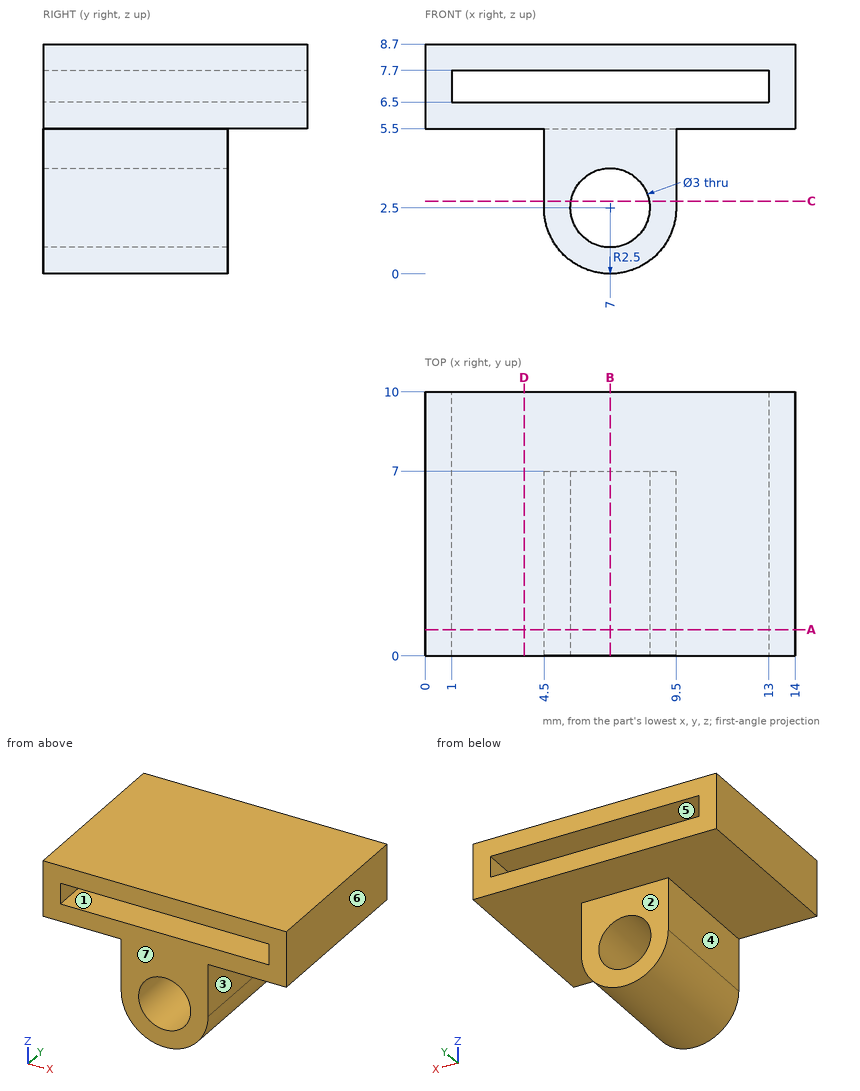
The figure shows three views and two pictorial views of one solid part (mm, origin at its lowest corner). Answer the questions. A direction names the side the tool comes from. Round coordinates to 2 decimals unless told otherwise and drop trailing zeros. Order: outer loops, then holes, each group sorted by start corner. A loop starts at its lowest first (then second) coordinate and runs counter-clockwise, first axis right, second up. Notation, with made-up numbers: (17.25, 56.25) -> (25.25, 56.25) arc R31 ccw to (25.25, 91.25) -> close; hole circle Ø8 at (-38.75, 84). An arc over 180 degrees is marked (long way). One line per item, written item: value.
Item 1: Find section A-A, the plane y = 1. Give the vertices of the cut face in (x, z), then the cut area to 3 significant figures.
Taken from the geometry:
outline: (0, 5.5) -> (4.5, 5.5) -> (4.5, 2.5) arc R2.5 ccw to (9.5, 2.5) -> (9.5, 5.5) -> (14, 5.5) -> (14, 8.7) -> (0, 8.7) -> close; hole (1, 6.5) -> (13, 6.5) -> (13, 7.7) -> (1, 7.7) -> close; hole circle Ø3 at (7, 2.5)
area: 48.1 mm2
Item 2: For the marked faces 1, 2, 3 and 4, determine the directions among +Z, -Z, +X, -X, +Y, -Y from which every point of the face is accessible in a straight line to the end or side of a thin tool.
Taken from the geometry:
face 1: +Y, -Y
face 2: -Z, +X, -X, +Y
face 3: -Z, +X, +Y, -Y
face 4: -Z, -X, +Y, -Y
Item 3: For a pull along X with two mould halves and no side action, classify the marked faces 5, 6 and 7 as released by +X, released by -X, zero draft, split by the parting line, or undercut.
Taken from the geometry:
face 5: undercut
face 6: released by +X
face 7: zero draft
Item 4: Find section C-C, the plane z = 2.75. Give the vertices of the cut face in (x, y), then the cut area to 3 significant figures.
Taken from the geometry:
outline: (4.5, 0) -> (5.52, 0) -> (5.52, 7) -> (4.5, 7) -> close; (8.48, 0) -> (9.5, 0) -> (9.5, 7) -> (8.48, 7) -> close
area: 14.3 mm2
Item 5: Given P1, Ø1.5, axis at y = 2, z = 4.5, coming from the -X side; P2, Ø3, axis at x = 4.5, y = 6, coming from the -Z side; P3, Ø2, axis at x = 9.5, y = 6, coming from the -Z side, each flat-ended and moving along its own axis, determine where each tip first touches the part or whether it passes through.
Taken from the geometry:
P1: stops at x = 4.5
P2: stops at z = 0.21
P3: stops at z = 0.5
Item 6: Find section B-B, the plane x = 7. Give the vertices of the cut face in (y, z), then the cut area to 3 significant figures.
Taken from the geometry:
outline: (0, 0) -> (7, 0) -> (7, 1) -> (0, 1) -> close; (0, 4) -> (7, 4) -> (7, 5.5) -> (10, 5.5) -> (10, 6.5) -> (0, 6.5) -> close; (0, 7.7) -> (10, 7.7) -> (10, 8.7) -> (0, 8.7) -> close
area: 37.5 mm2
Item 7: Straight lines are drawn through the part: L1, parallel to X at y = 3.75, z = 2.5; L2, parallel to Z at x = 11.75, y = 4.25; L3, parallel to Z at x = 8, y = 5.5. For each, find the intervals that lie inside material, in ascending order.
Taken from the geometry:
L1: x = 4.5 to 5.5, 8.5 to 9.5
L2: z = 5.5 to 6.5, 7.7 to 8.7
L3: z = 0.21 to 1.38, 3.62 to 6.5, 7.7 to 8.7
Item 8: Find section D-D, the plane x = 3.75. Give the vertices of the cut face in (y, z).
Taken from the geometry:
outline: (0, 5.5) -> (10, 5.5) -> (10, 6.5) -> (0, 6.5) -> close; (0, 7.7) -> (10, 7.7) -> (10, 8.7) -> (0, 8.7) -> close
